```python
from build123d import *

# Parameters (mm, degrees)
BOSS_EXTRUDE1_DEPTH = 3
BOSS_EXTRUDE2_DEPTH = 15.1


with BuildPart() as part:
    # Sketch1 → Boss-Extrude1 (new body)
    with BuildSketch(Plane(origin=(0, 0, 0), x_dir=(1, 0, 0), z_dir=(0, 1, 0))):
        Polygon((2, 0), (2, -5), (-3, -5), (-3, -23.9), (23.2, -23.9), (23.2, -5), (18.2, -5), (18.2, 0), align=None)
    extrude(amount=BOSS_EXTRUDE1_DEPTH)

    # Sketch1<3> → Boss-Extrude2 (add)
    with BuildSketch(Plane(origin=(0, 0, 0), x_dir=(1, 0, 0), z_dir=(0, 1, 0))):
        Polygon((5, -8), (5, 0), (2, 0), (2, -5), (-3, -5), (-3, -23.9), (0, -23.9), (0, -8), align=None)
        Polygon((18.2, 0), (15.2, 0), (15.2, -8), (20.2, -8), (20.2, -23.9), (23.2, -23.9), (23.2, -5), (18.2, -5), align=None)
    extrude(amount=BOSS_EXTRUDE2_DEPTH)


solid = part.part
```
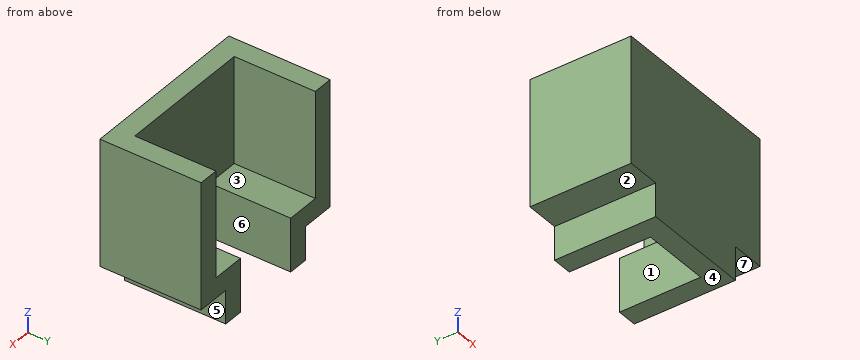
Check sheet for the modelled part. Datum: model origin and axes. Units: mm. Face numbers are marked on the shaded views. A direction names the side the tool comes from. Round coordinates to 2 decimals unless told otherwise and drop trailing zeros. Loops run counter-clockwise (first coordinate to the right, second up) from the corner with the lowest first, then second, coordinate; pieces in that order, holes last. Notation, with made-up numbers: (39, 9.5) - (67, 9.5) arc R20 cw to (67, 22.5) - close; hole circle Ø2 at (-16, 28). An arc over 180 degrees is marked (long way). Write item = value, one per line. Start each with the question number.
Q1. Section check C-C (y = 1.5). Record the boundary of the cut face in (x, z).
Q2. Depth check by flat-ended pin: P1, Ø5, axis at x = 19.5, y = 2, coming from the -Z side; P2, Ø5.5, axis at y = 6, z = 2, coming from the +X side; P3, Ø4, axis at x = 21, y = 10.5, coming from the -Z side; P4, Ø1.5, axis at x = 17, y = 9, coming from the +Z side. Enter the tip coordinate at first touch or a pass-through.
Q3. Section check A-A (y = 8.5). Record the boundary of the cut face in (x, z).
Q4. Section check B-B (z = 17.25). Record the boundary of the cut face in (x, y).
Q5. Thickness scan on L1, parallel to X at y = 5.75, z = 21; L2, parallel to X at y = 12.25, z = 7.5; L3, parallel to Y at x = 13.5, z = 4.75. Record the ranges inside material, lowest first.
Q6. Access from +Z, -Z, +X, -X, +Y, -Y to the whole of each face (thin tool, end or side, straight path). Record for the marked faces 1, 2, 3 and 4.
Q7. Section check D-D (x = 12). Record the boundary of the cut face in (y, z).
Q8. Release check for a two-part mould opening along X. For the marked faces 5, 6 and 7 record: pulls with the +X half, pulls with the -X half, needs draft (parallel to the pull), parting line crosses it, or undercut.
Derived:
q1.outline = (-3, 5) - (2, 5) - (2, 0) - (18.2, 0) - (18.2, 5) - (23.2, 5) - (23.2, 23.9) - (-3, 23.9) - close
q2.P1 = 0
q2.P2 = 18.2
q2.P3 = 5
q2.P4 = 8
q3.outline = (-3, 5) - (2, 5) - (2, 0) - (5, 0) - (5, 8) - (0, 8) - (0, 23.9) - (-3, 23.9) - close; (15.2, 0) - (18.2, 0) - (18.2, 5) - (23.2, 5) - (23.2, 23.9) - (20.2, 23.9) - (20.2, 8) - (15.2, 8) - close
q4.outline = (-3, 0) - (23.2, 0) - (23.2, 15.1) - (20.2, 15.1) - (20.2, 3) - (0, 3) - (0, 15.1) - (-3, 15.1) - close
q5.L1 = -3 to 0, 20.2 to 23.2
q5.L2 = -3 to 5, 15.2 to 23.2
q5.L3 = 0 to 3
q6.face_1 = +Z, -Z, +Y
q6.face_2 = -Z, -X, +Y, -Y
q6.face_3 = +Z, +Y
q6.face_4 = -Z, +X, -X, +Y, -Y
q7.outline = (0, 0) - (3, 0) - (3, 23.9) - (0, 23.9) - close
q8.face_5 = pulls with the +X half
q8.face_6 = undercut
q8.face_7 = needs draft
